Autodesk Inventor part; units mm, degrees
ref_plane "YZ Plane" through (0, 0, 0) normal (1, 0, 0) x (0, 1, 0)
ref_plane "XZ Plane" through (0, 0, 0) normal (0, 1, 0) x (-1, 0, 0)
ref_plane "XY Plane" through (0, 0, 0) normal (0, 0, 1) x (1, 0, 0)
sketch "Sketch1" plane through (0, 0, 0) normal (0, 0, 1) x (1, 0, 0)
  line L0 (0, 0) -> (0, 12.4297) construction
  line L1 (7.987, 0) -> (9.9363, 0)
  line L2 (9.9363, 0) -> (12.195, 2.2587)
  line L3 (12.195, 2.2587) -> (9.3387, 5.115)
  line L4 (9.3387, 5.115) -> (12.195, 7.9713)
  line L5 (12.195, 7.9713) -> (9.9363, 10.23)
  line L6 (9.9363, 10.23) -> (7.987, 10.23)
  line L7 (7.987, 10.23) -> (7.987, 0)
  line L8 (7.987, 5.115) -> (38.026, 5.115) construction
  line L9 (0, 0) -> (31.3179, 0) construction
  dimension "d0" = 10.23
  dimension "d1" = 15.974
  dimension "d2" = 90
  dimension "d4" = 90
  dimension "d5" = 24.39
revolve "Revolution1" add sketch "Sketch1" angle 360 about axis through (0, 0, 0) along (0, 1, 0)
properties part number "Delrin V-Wheel"
For this review, take the finished solid that the model builds, in its own axes (mm). A direction names the side the tool comes from. Coordinates: 2 decimals unless noted, no trailing zeros. Write each loop counter-clockwise with the first axis right and the second up, starting at its lowest first coordinate (ties: lowest second). Pieces come first, ordered by that corner, then holes. Notation, with made-up numbers: (-37, -9) -> (-16, -9) arc R33 cw to (-16, 30) -> close; hole circle Ø4 at (65, -21.75). An arc over 180 degrees is marked (long way). Write each question's results on one line, items separated by ' | '. Start each with the question number.
1) For faces 1 (the face through (9.61, 10.09, 3.03)), 2 (the face through (-2.06, 5.29, 9.29)), list the 3-axis set-ups (+Z, -Z, +X, -X, +Y, -Y) from which the entire face can be reached by the end or side of a thin tool; tool diameter is ignored.
2) Consider section D-D (y = 6.5). Write out the cut boundary in (x, z), plus the area to 3 significant figures.
3) Consider section C-C (y = 4). Write out the cut boundary in (x, z), plus the area to 3 significant figures.
4) Consider section A-A (z = 0). Write out the cut boundary in (x, y) (3 decimals).
5) Wall thickness on L1, parallel to X at y = 7, z = 0.75; L2, parallel to Y at x = 4.5, z = 8.75; L3, parallel to Y at x = -7, z = -7: over which ranges is each line inside the solid? List them lowest first. Write a range as [from, to].
6) Consider section B-B (x = 0). Write out the cut boundary in (y, z) (3 decimals).
7) Insertion check: pin 1 (4 mm diameter, centred on y = 6.5, z = 8, fed in from +X); pin 2 (14.5 mm diameter, centred on x = 0, z = 0, fed in from -Y); pin 3 (1.5 mm diameter, centred on x = -8.5, z = -8, fed in from +Y). Each pin has a flat end and moves straight along its axis. Give the tip position at first contact, or say it passes through.
8) The part is to be moulded in two halves that separate along Z. For faces 3 (the face through (-1.239, 4.936, 9.436)), 4 (the face through (-5.887, 5.043, 5.398)), 5 (the face through (-0.05, 0, -8.14)), say which applies: +Z half, -Z half, draft (parallel to the pull), parting line (faces both ways), or undercut.
Geometry says:
1) face 1: +Y | face 2: none
2) outline: circle Ø21.45 at (0, 0); hole circle Ø15.97 at (0, 0) | area: 161 mm^2
3) outline: circle Ø20.91 at (0, 0); hole circle Ø15.97 at (0, 0) | area: 143 mm^2
4) outline: (-12.195, 2.259) -> (-9.936, 0) -> (-7.987, 0) -> (-7.987, 10.23) -> (-9.936, 10.23) -> (-12.195, 7.971) -> (-9.339, 5.115) -> close; (7.987, 0) -> (9.936, 0) -> (12.195, 2.259) -> (9.339, 5.115) -> (12.195, 7.971) -> (9.936, 10.23) -> (7.987, 10.23) -> close
5) L1: [-11.2, -7.95], [7.95, 11.2] | L2: [0, 4.61], [5.62, 10.23] | L3: [0, 4.55], [5.68, 10.23]
6) outline: (0, -9.936) -> (2.259, -12.195) -> (5.115, -9.339) -> (7.971, -12.195) -> (10.23, -9.936) -> (10.23, -7.987) -> (0, -7.987) -> close; (0, 7.987) -> (10.23, 7.987) -> (10.23, 9.936) -> (7.971, 12.195) -> (5.115, 9.339) -> (2.259, 12.195) -> (0, 9.936) -> close
7) pin 1: x = 10.23 | pin 2: through | pin 3: y = 9.24
8) face 3: parting line | face 4: undercut | face 5: draft
